from build123d import *

# Parameters (mm, degrees)
SKETCH_2_W          = 31
SKETCH_2_H          = 25
EXTRUDE_1_DEPTH     = 3
SKETCH_3_W          = 31
SKETCH_3_H          = 1
CUT_EXTRUDE_1_DEPTH = 2.5
SKETCH_4_W          = 5
SKETCH_4_H          = 22
CUT_EXTRUDE_2_DEPTH = 2.5
FILLET_11_R         = 1
FILLET_12_R         = 1
FILLET_13_R         = 1
FILLET_18_R         = 1
FILLET_19_R         = 1
FILLET_20_R         = 1
FILLET_21_R         = 1
FILLET_22_R         = 0.2
FILLET_23_R         = 0.2
FILLET_24_R         = 0.2


# Some blends are built 0.0001 mm under size
with BuildPart() as part:
    # 草图2 → 凸台-拉伸1 (new body)
    with BuildSketch(Plane(origin=(0, 0, 0), x_dir=(1, 0, 0), z_dir=(0, 1, 0))):
        Rectangle(SKETCH_2_W, SKETCH_2_H)
    extrude(amount=EXTRUDE_1_DEPTH)

    # 草图3 → 切除-拉伸1 (cut)
    with BuildSketch(Plane(origin=(0, 3, 0), x_dir=(1, 0, 0), z_dir=(0, 1, 0))):
        with Locations((0, 11.5)):
            Rectangle(SKETCH_3_W, SKETCH_3_H)
        with Locations((0, -11.5)):
            Rectangle(SKETCH_3_W, SKETCH_3_H)
    extrude(amount=-CUT_EXTRUDE_1_DEPTH, mode=Mode.SUBTRACT)

    # 草图4 → 切除-拉伸2 (cut)
    with BuildSketch(Plane(origin=(0, 3, 0), x_dir=(1, 0, 0), z_dir=(0, 1, 0))):
        with Locations((-13, 0)):
            Rectangle(SKETCH_4_W, SKETCH_4_H)
    extrude(amount=-CUT_EXTRUDE_2_DEPTH, mode=Mode.SUBTRACT)

    # 圆角11
    fillet_11_edges = [part.edges().sort_by_distance(p)[0] for p in [
        (0, 0, 12.5),
    ]]
    fillet(fillet_11_edges, radius=FILLET_11_R)

    # 圆角12
    fillet_12_edges = [part.edges().sort_by_distance(p)[0] for p in [
        (0, 0, -12.5),
    ]]
    fillet(fillet_12_edges, radius=FILLET_12_R)

    # 圆角13
    # the kernel refuses this fillet: 1 mm, written as the material it takes off along each edge
    with BuildSketch(Plane(origin=(15.5, 1, 12.5), x_dir=(0, 0, -1), z_dir=(0, 1, 0))) as fillet_13_piece_1:
        with BuildLine():
            CenterArc((FILLET_13_R, FILLET_13_R), FILLET_13_R, 180, 90)
            Line((0, FILLET_13_R), (0, 0))
            Line((0, 0), (FILLET_13_R, 0))
        make_face()
    extrude(amount=4.5, mode=Mode.SUBTRACT)
    with BuildSketch(Plane(origin=(15.5, 1, -12.5), x_dir=(0, 0, 1), z_dir=(0, 1, 0))) as fillet_13_piece_2:
        with BuildLine():
            CenterArc((FILLET_13_R, -FILLET_13_R), FILLET_13_R, 90, 90)
            Line((0, -FILLET_13_R), (0, 0))
            Line((0, 0), (FILLET_13_R, 0))
        make_face()
    extrude(amount=4.5, mode=Mode.SUBTRACT)
    with BuildSketch(Plane(origin=(15.5, 0, -11.5), x_dir=(0, 1, 0), z_dir=(0, 0, 1))) as fillet_13_piece_3:
        with BuildLine():
            CenterArc((FILLET_13_R, FILLET_13_R), FILLET_13_R, 180, 90)
            Line((0, FILLET_13_R), (0, 0))
            Line((0, 0), (FILLET_13_R, 0))
        make_face()
    extrude(amount=23, mode=Mode.SUBTRACT)
    with BuildSketch(Plane(origin=(15.5, 1, -11.5), x_dir=(0, -1, 0), z_dir=(0, 0, 1))) as fillet_13_piece_4:
        with BuildLine():
            CenterArc((1 - FILLET_13_R, -FILLET_13_R), FILLET_13_R, 0, 90)
            Line((1, -FILLET_13_R), (1, 0))
            Line((1, 0), (1 - FILLET_13_R, 0))
        make_face()
    revolve(axis=Axis((15.5, 1, -11.5), (1, 0, 0)), revolution_arc=90, mode=Mode.SUBTRACT)
    with BuildSketch(Plane(origin=(15.5, 1, 11.5), x_dir=(0, 0, 1), z_dir=(0, 1, 0))) as fillet_13_piece_5:
        with BuildLine():
            CenterArc((1 - FILLET_13_R, -FILLET_13_R), FILLET_13_R, 0, 90)
            Line((1, -FILLET_13_R), (1, 0))
            Line((1, 0), (1 - FILLET_13_R, 0))
        make_face()
    revolve(axis=Axis((15.5, 1, 11.5), (1, 0, 0)), revolution_arc=90, mode=Mode.SUBTRACT)

    # 圆角18
    fillet_18_edges = [part.edges().sort_by_distance(p)[0] for p in [
        (15.5, 3, 0),
        (2.5, 3, 11),
        (2.5, 3, -11),
        (-10.5, 3, 0),
    ]]
    fillet(fillet_18_edges, radius=FILLET_18_R)

    # 圆角19
    fillet_19_edges = [part.edges().sort_by_distance(p)[0] for p in [
        (-10.5, 0.5, 0),
    ]]
    fillet(fillet_19_edges, radius=FILLET_19_R)

    # 圆角20
    fillet_20_edges = [part.edges().sort_by_distance(p)[0] for p in [
        (1.933012702, 0.5, -11),
    ]]
    fillet(fillet_20_edges, radius=FILLET_20_R - 0.0001)  # a hair under: the kernel refuses the full size

    # 圆角21
    fillet_21_edges = [part.edges().sort_by_distance(p)[0] for p in [
        (1.933012702, 0.5, 11),
    ]]
    fillet(fillet_21_edges, radius=FILLET_21_R - 0.0001)  # a hair under: the kernel refuses the full size

    # 圆角22
    fillet_22_edges = [part.edges().sort_by_distance(p)[0] for p in [
        (-15.5, 3, 12.25),
        (-0.5, 3, 12.5),
        (-0.066987298, 3, 12),
        (15, 3, 12.366025404),
    ]]
    fillet(fillet_22_edges, radius=FILLET_22_R)

    # 圆角23
    fillet_23_edges = [part.edges().sort_by_distance(p)[0] for p in [
        (-15.5, 3, -12.25),
        (-0.5, 3, -12.5),
        (-0.066987298, 3, -12),
        (15, 3, -12.366025404),
    ]]
    fillet(fillet_23_edges, radius=FILLET_23_R)

    # 圆角24
    # the kernel refuses this fillet: 0.2 mm, written as the material it takes off along each edge
    with BuildSketch(Plane(origin=(-15.3, 2.8, 12.2), x_dir=(0, 0, -1), z_dir=(-1, 0, 0))) as fillet_24_piece_1_section:
        Polygon((0, 0), (FILLET_24_R, 0), (FILLET_24_R, -FILLET_24_R), (0, -FILLET_24_R), align=None)
    fillet_24_piece_1 = extrude(amount=FILLET_24_R, mode=Mode.PRIVATE)
    fillet_24_piece_1 = fillet_24_piece_1 - Plane(origin=(-15.3, 2.8, 12.2), x_dir=(0, -0.7071067811865475, 0.7071067811865475), z_dir=(-1, 0, 0)) * Sphere(FILLET_24_R, mode=Mode.PRIVATE)
    add(fillet_24_piece_1, mode=Mode.SUBTRACT)
    with BuildSketch(Plane(origin=(-15.3, 2.8, 12.3), x_dir=(0, 0, 1), z_dir=(-1, 0, 0))) as fillet_24_piece_2_section:
        Polygon((0, 0), (FILLET_24_R, 0), (FILLET_24_R, FILLET_24_R), (0, FILLET_24_R), align=None)
    fillet_24_piece_2 = extrude(amount=FILLET_24_R, mode=Mode.PRIVATE)
    fillet_24_piece_2 = fillet_24_piece_2 - Plane(origin=(-15.3, 2.8, 12.3), x_dir=(0, -0.7071067811865475, -0.7071067811865475), z_dir=(-1, 0, 0)) * Sphere(FILLET_24_R, mode=Mode.PRIVATE)
    add(fillet_24_piece_2, mode=Mode.SUBTRACT)
    with BuildSketch(Plane(origin=(-15.3, 2.8, -12.3), x_dir=(0, 0, -1), z_dir=(-1, 0, 0))) as fillet_24_piece_3_section:
        Polygon((0, 0), (FILLET_24_R, 0), (FILLET_24_R, -FILLET_24_R), (0, -FILLET_24_R), align=None)
    fillet_24_piece_3 = extrude(amount=FILLET_24_R, mode=Mode.PRIVATE)
    fillet_24_piece_3 = fillet_24_piece_3 - Plane(origin=(-15.3, 2.8, -12.3), x_dir=(0, -0.7071067811865475, 0.7071067811865475), z_dir=(-1, 0, 0)) * Sphere(FILLET_24_R, mode=Mode.PRIVATE)
    add(fillet_24_piece_3, mode=Mode.SUBTRACT)
    with BuildSketch(Plane(origin=(-15.3, 2.8, -12.2), x_dir=(0, 0, 1), z_dir=(-1, 0, 0))) as fillet_24_piece_4_section:
        Polygon((0, 0), (FILLET_24_R, 0), (FILLET_24_R, FILLET_24_R), (0, FILLET_24_R), align=None)
    fillet_24_piece_4 = extrude(amount=FILLET_24_R, mode=Mode.PRIVATE)
    fillet_24_piece_4 = fillet_24_piece_4 - Plane(origin=(-15.3, 2.8, -12.2), x_dir=(0, -0.7071067811865475, -0.7071067811865475), z_dir=(-1, 0, 0)) * Sphere(FILLET_24_R, mode=Mode.PRIVATE)
    add(fillet_24_piece_4, mode=Mode.SUBTRACT)
    with BuildSketch(Plane(origin=(-15.5, 1, 12.5), x_dir=(0, 0, -1), z_dir=(0, 1, 0))) as fillet_24_piece_5:
        with BuildLine():
            CenterArc((FILLET_24_R, -FILLET_24_R), FILLET_24_R, 90, 90)
            Line((0, -FILLET_24_R), (0, 0))
            Line((0, 0), (FILLET_24_R, 0))
        make_face()
    extrude(amount=1.8, mode=Mode.SUBTRACT)
    with BuildSketch(Plane(origin=(-15.5, 1, -12.5), x_dir=(0, 0, 1), z_dir=(0, 1, 0))) as fillet_24_piece_6:
        with BuildLine():
            CenterArc((FILLET_24_R, FILLET_24_R), FILLET_24_R, 180, 90)
            Line((0, FILLET_24_R), (0, 0))
            Line((0, 0), (FILLET_24_R, 0))
        make_face()
    extrude(amount=1.8, mode=Mode.SUBTRACT)
    with BuildSketch(Plane(origin=(-15.5, 0.5, 12), x_dir=(0, -1, 0), z_dir=(0, 0, -1))) as fillet_24_piece_7:
        with BuildLine():
            CenterArc((FILLET_24_R, -FILLET_24_R), FILLET_24_R, 90, 90)
            Line((0, -FILLET_24_R), (0, 0))
            Line((0, 0), (FILLET_24_R, 0))
        make_face()
    extrude(amount=24, mode=Mode.SUBTRACT)
    with BuildSketch(Plane(origin=(-15.5, 2.8, -12), x_dir=(0, 0, -1), z_dir=(0, -1, 0))) as fillet_24_piece_8:
        with BuildLine():
            CenterArc((FILLET_24_R, FILLET_24_R), FILLET_24_R, 180, 90)
            Line((0, FILLET_24_R), (0, 0))
            Line((0, 0), (FILLET_24_R, 0))
        make_face()
    extrude(amount=2.3, mode=Mode.SUBTRACT)
    with BuildSketch(Plane(origin=(-15.5, 2.8, 12), x_dir=(0, 0, 1), z_dir=(0, -1, 0))) as fillet_24_piece_9:
        with BuildLine():
            CenterArc((FILLET_24_R, -FILLET_24_R), FILLET_24_R, 90, 90)
            Line((0, -FILLET_24_R), (0, 0))
            Line((0, 0), (FILLET_24_R, 0))
        make_face()
    extrude(amount=2.3, mode=Mode.SUBTRACT)
    with BuildSketch(Plane(origin=(-15.5, 1, 11.5), x_dir=(0, 0, 1), z_dir=(0, 1, 0))) as fillet_24_piece_10:
        with BuildLine():
            CenterArc((1 - FILLET_24_R, FILLET_24_R), FILLET_24_R, 270, 90)
            Line((1, FILLET_24_R), (1, 0))
            Line((1, 0), (1 - FILLET_24_R, 0))
        make_face()
    revolve(axis=Axis((-15.5, 1, 11.5), (1, 0, 0)), revolution_arc=90, mode=Mode.SUBTRACT)
    with BuildSketch(Plane(origin=(-15.5, 0, 11.5), x_dir=(0, 1, 0), z_dir=(0, 0, -1))) as fillet_24_piece_11:
        with BuildLine():
            CenterArc((FILLET_24_R, FILLET_24_R), FILLET_24_R, 180, 90)
            Line((0, FILLET_24_R), (0, 0))
            Line((0, 0), (FILLET_24_R, 0))
        make_face()
    extrude(amount=23, mode=Mode.SUBTRACT)
    with BuildSketch(Plane(origin=(-15.5, 1, -11.5), x_dir=(0, -1, 0), z_dir=(0, 0, 1))) as fillet_24_piece_12:
        with BuildLine():
            CenterArc((1 - FILLET_24_R, FILLET_24_R), FILLET_24_R, 270, 90)
            Line((1, FILLET_24_R), (1, 0))
            Line((1, 0), (1 - FILLET_24_R, 0))
        make_face()
    revolve(axis=Axis((-15.5, 1, -11.5), (1, 0, 0)), revolution_arc=90, mode=Mode.SUBTRACT)
    with BuildSketch(Plane(origin=(-15.5, 0.5, 12.5), x_dir=(0, -1, 0), z_dir=(0, 0, -1))) as fillet_24_piece_13a_section:
        with BuildLine():
            CenterArc((FILLET_24_R, -FILLET_24_R), FILLET_24_R, 90, 90)
            Line((0, -FILLET_24_R), (0, 0))
            Line((0, 0), (FILLET_24_R, 0))
        make_face()
    fillet_24_piece_13a = extrude(amount=24.5, mode=Mode.PRIVATE)
    fillet_24_piece_13a = split(fillet_24_piece_13a, bisect_by=Plane(origin=(-15.454720977, 0.454720977, 12), z_dir=(0, 0, 1)), keep=Keep.TOP, mode=Mode.PRIVATE)
    with BuildSketch(Plane(origin=(-15.5, 2.8, 12), x_dir=(0, 0, 1), z_dir=(0, -1, 0))) as fillet_24_piece_13b_section:
        with BuildLine():
            CenterArc((FILLET_24_R, -FILLET_24_R), FILLET_24_R, 90, 90)
            Line((0, -FILLET_24_R), (0, 0))
            Line((0, 0), (FILLET_24_R, 0))
        make_face()
    fillet_24_piece_13b = extrude(amount=2.8, mode=Mode.PRIVATE)
    fillet_24_piece_13b = split(fillet_24_piece_13b, bisect_by=Plane(origin=(-15.454720977, 0.5, 12.045279023), z_dir=(0, -1, 0)), keep=Keep.TOP, mode=Mode.PRIVATE)
    fillet_24_piece_13 = fillet_24_piece_13a & fillet_24_piece_13b
    add(fillet_24_piece_13, mode=Mode.SUBTRACT)
    with BuildSketch(Plane(origin=(-15.5, 2.8, -12), x_dir=(0, 0, -1), z_dir=(0, -1, 0))) as fillet_24_piece_14a_section:
        with BuildLine():
            CenterArc((FILLET_24_R, FILLET_24_R), FILLET_24_R, 180, 90)
            Line((0, FILLET_24_R), (0, 0))
            Line((0, 0), (FILLET_24_R, 0))
        make_face()
    fillet_24_piece_14a = extrude(amount=2.8, mode=Mode.PRIVATE)
    fillet_24_piece_14a = split(fillet_24_piece_14a, bisect_by=Plane(origin=(-15.454720977, 0.5, -12.045279023), z_dir=(0, -1, 0)), keep=Keep.TOP, mode=Mode.PRIVATE)
    with BuildSketch(Plane(origin=(-15.5, 0.5, 12), x_dir=(0, -1, 0), z_dir=(0, 0, -1))) as fillet_24_piece_14b_section:
        with BuildLine():
            CenterArc((FILLET_24_R, -FILLET_24_R), FILLET_24_R, 90, 90)
            Line((0, -FILLET_24_R), (0, 0))
            Line((0, 0), (FILLET_24_R, 0))
        make_face()
    fillet_24_piece_14b = extrude(amount=24.5, mode=Mode.PRIVATE)
    fillet_24_piece_14b = split(fillet_24_piece_14b, bisect_by=Plane(origin=(-15.454720977, 0.454720977, -12), z_dir=(0, 0, -1)), keep=Keep.TOP, mode=Mode.PRIVATE)
    fillet_24_piece_14 = fillet_24_piece_14a & fillet_24_piece_14b
    add(fillet_24_piece_14, mode=Mode.SUBTRACT)


solid = part.part
Geometry: final body of the model. Coordinates: model frame, mm. A direction names the side the tool comes from. Round coordinates to 2 decimals unless told otherwise and drop trailing zeros. Loops run counter-clockwise (first coordinate to the right, second up) from the corner with the lowest first, then second, coordinate; pieces in that order, holes last. Notation, with made-up numbers: M 11.5,16.25 L 22.5,16.25 A7 ccw 22.5,22.25 Z; hole C 64,68 d7. An arc over 180 degrees is marked long. Put each result on its own line as item: value. Start each with the question number.
(1) Draft query along Z for faces 5 (the face through (15.5, 1.5, 0.2)), 6 (the face through (-0.191, 0.285, -12.199)), 7 (the face through (1.811, 0.801, -11.285)), 8 (the face through (-10.785, 0.801, -0.168)). Return one class per face: +Z half, -Z half, draft (parallel to the pull), parting line (faces both ways), or undercut.
(2) Material intervals for line 1 along Z through (x, y) = (-8, 1.95); line 2 along Z through (x, y) = (11, 2.45); line 3 along Z through (x, y) = (-14, 1.9), sorted ascending. Write a range as [from, to].
(3) Section query A-A (z = -8.75). Return loops of the section in (x, y), then the cut area to 3 significant figures.
(4) Set-up query: faces 1 (the face through (15.199, 0.285, -0.161)), 2 (the face through (2.682, 2.699, 10.715)), 3 (the face through (15.215, 2.699, -0.154)), 4 (the face through (-10.215, 2.699, -0.154)). Return all of +Z, -Z, +X, -X, +Y, -Y with unobstructed straight access to the full face (end or side cutting, diameter ignored); none if empty.
(5) Contact query for a flat-ended pin moving along its axis: pin 1 Ø1 at (y, z) = (1.5, -5) entering from -X. Output: stop coordinate, or through.
Findings below:
1. face 5: draft
1. face 6: -Z half
1. face 7: undercut
1. face 8: undercut
2. line 1: z = [-12.5, -12], [-11, 11], [12, 12.5]
2. line 2: z = [-12.5, -12], [-10.89, 10.89], [12, 12.5]
2. line 3: z = [-12.5, -12], [12, 12.5]
3. outline: M -15.5,0.2 A0.2 ccw -15.3,0 L 14.5,0 A1 ccw 15.5,1 L 15.5,2 A1 ccw 14.5,3 L -9.5,3 A1 ccw -10.5,2 L -10.5,1.5 A1 cw -11.5,0.5 L -15.3,0.5 A0.2 ccw -15.5,0.3 Z
3. area: 80.1 mm2
4. face 1: +Z, -Z, +X, -Y
4. face 2: +X, -X, +Y
4. face 3: +X, +Y
4. face 4: -X, +Y
5. pin 1: stops at x = -10.63
